from build123d import *

# Parameters (mm, degrees)
SKETCH_1_R      = 7
EXTRUDE_1_DEPTH = 8
SKETCH_2_R      = 7
SKETCH_2_R_2    = 2.5
EXTRUDE_2_DEPTH = 10


with BuildPart() as part:
    # Эскиз1 → Бобышка-Вытянуть1 (new body)
    with BuildSketch(Plane.XY):
        Circle(SKETCH_1_R)
        Polygon((2.280533563, -3.95), (4.561067127, 0), (2.280533563, 3.95), (-2.280533563, 3.95), (-4.561067127, 0), (-2.280533563, -3.95), align=None, mode=Mode.SUBTRACT)
    extrude(amount=EXTRUDE_1_DEPTH)

    # Эскиз2 → Бобышка-Вытянуть2 (add)
    with BuildSketch(Plane.XY.offset(8)):
        Circle(SKETCH_2_R)
        Circle(SKETCH_2_R_2, mode=Mode.SUBTRACT)
    extrude(amount=EXTRUDE_2_DEPTH)


solid = part.part
Could you check a few things on this model? Use its own coordinates, in mm. A direction names the side the tool comes from. Coordinates: 2 decimals unless noted, no trailing zeros. Write each loop counter-clockwise with the first axis right and the second up, starting at its lowest first coordinate (ties: lowest second). Pieces come first, ordered by that corner, then holes. Notation, with made-up numbers: M 51.25,0 L 102.25,0 A23 ccw 102.25,17 Z; hole C 80,82.5 d1. An arc over 180 degrees is marked long. One line per question, with ' | ' between items.
1) Imagine slicing it at C-C, the plane y = -2.25. Write out the boundary of the cut face in (x, z), and give its area (3 significant figures).
Checks:
outline: M -6.63,0 L -3.26,0 L -3.26,8 L -1.09,8 L -1.09,18 L -6.63,18 Z; M 1.09,8 L 3.26,8 L 3.26,0 L 6.63,0 L 6.63,18 L 1.09,18 Z | area: 165 mm²
2) Imagine slicing it at D-D, the plane x = 3.75. Write out the boundary of the cut face in (y, z), and give its area (3 significant figures).
Checks:
outline: M -5.91,0 L -1.4,0 L -1.4,8 L 1.4,8 L 1.4,0 L 5.91,0 L 5.91,18 L -5.91,18 Z | area: 190 mm²
3) For pin 1 Ø6.5 at (x, y) = (0, 0) entering from -Z; pin 2 Ø1 at (x, z) = (5.5, 11) entering from -Y; pin 3 Ø1.5 at (x, z) = (-3, 10.5) entering from +Y, each with a flat end and sliding along its axis, tell me the tip position at first contact or that it passes through.
Checks:
pin 1: z = 8 | pin 2: y = -4.9 | pin 3: y = 6.63
4) Imagine slicing it at B-B, the plane z = 5.5. Write out the boundary of the cut face in (x, y).
Checks:
outline: C 0,0 d14; hole M -4.56,0 L -2.28,-3.95 L 2.28,-3.95 L 4.56,0 L 2.28,3.95 L -2.28,3.95 Z
5) If we mould it in two halves opening along X, with no side actions, what happens to faces 1 (the face through (0, -3, 18)), 2 (the face through (6.466, -2.681, 8.874)), 3 (the face through (2, 2, 8)), 4 (the face through (0, 3.95, 4))? For each: released by +X, released by -X, zero draft, split by the parting line, or undercut.
Checks:
face 1: zero draft | face 2: split by the parting line | face 3: undercut | face 4: undercut
6) I need wall thicknesses on probe 1 along Y at (x, z) = (0, 9); probe 2 along Z at (x, y) = (2.5, 1.75); probe 3 along X at (y, z) = (1.25, 11.5). Which ranges of each line are inside material? Lowest first, please. Write a range as [from, to].
Checks:
probe 1: [-7, -2.5], [2.5, 7] | probe 2: [8, 18] | probe 3: [-6.89, -2.17], [2.17, 6.89]
7) For faces 5 (the face through (3.405, -2.003, 3.944)), 6 (the face through (3.01, -3.01, 0)), which set-ups out of +Z, -Z, +X, -X, +Y, -Y let a thin tool reach every point of the face, with its end or its side?
Checks:
face 5: -Z | face 6: -Z, +X, -X, +Y, -Y
8) Imagine slicing it at A-A, the plane x = 0. Write out the boundary of the cut face in (y, z), and give its area (3 significant figures).
Checks:
outline: M -7,0 L -3.95,0 L -3.95,8 L -2.5,8 L -2.5,18 L -7,18 Z; M 2.5,8 L 3.95,8 L 3.95,0 L 7,0 L 7,18 L 2.5,18 Z | area: 139 mm²
